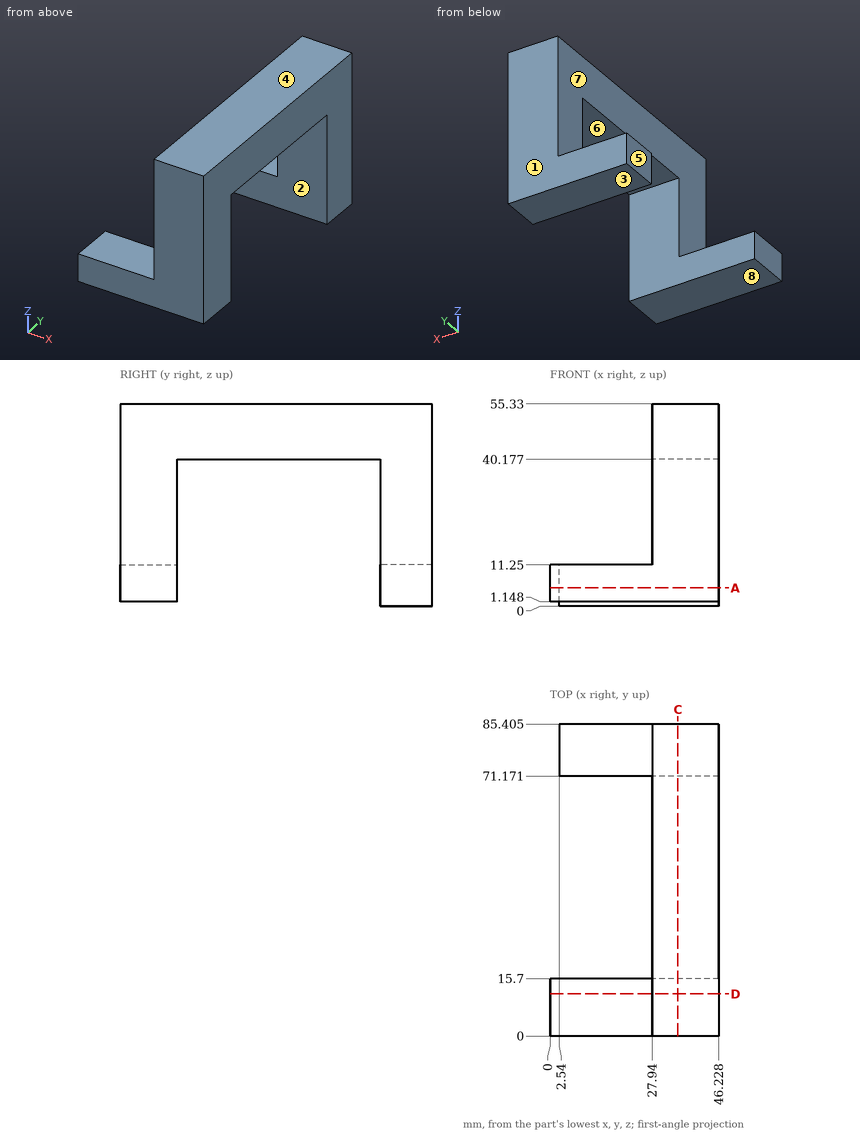
Job drawing, mm, ordinate dimensions from the low corner. One solid piece. A direction names the side the tool comes from. Coordinates: 2 decimals unless noted, no trailing zeros. Loops run counter-clockwise (first coordinate to the right, second up) from the corner with the lowest first, then second, coordinate; pieces in that order, holes last. Notation, with made-up numbers: (48.25, 85) - (89.25, 85) arc R22 cw to (89.25, 102) - close; hole circle Ø3 at (36.25, 69.5). An arc over 180 degrees is marked (long way). Write item = value, one per line. Start each with the question number.
Q1. Cut at A-A, the plane z = 5. List the corners of the cut face in (x, y) (1 decimal), then the cut area to 3 significant figures.
Q2. Cut at D-D, the plane y = 11.5. List the corners of the cut face in (x, z), then the cut area to 3 significant figures.
Q3. Which spindle directions (+Z, -Z, +X, -X, +Y, -Y) get a long thin tool onto all of the face, cutting with end or side? Do the marked faces 4, 5, 6, 7 and 8. Say none if no direction does.
Q4. Cut at C-C, the plane x = 35. List the corners of the cut face in (y, z) (1 decimal).
Q5. Flat gauge pins, fed straight in: pin 1 Ø12.5 at (x, y) = (18.5, 4) entering from -Z; pin 2 Ø5.5 at (x, y) = (40, 51) entering from -Z; pin 3 Ø15.5 at (x, y) = (14.5, 79) entering from +Z. Where does each tip first touch, or does it go through?
Q6. Drill centre lines: L1, parallel to Y at x = 40.5, z = 23.5 (1 decimal); L2, parallel to X at y = 14.5, z = 45; L3, parallel to Z at x = 23.5, y = 8.5. Where is each one in solid material? Low to high.
Q7. Pull direction Y, two halves, no side cores. Call the marked faces 1, 2 and 3: pulls with the +Y half, pulls with the -Y half, needs draft (parallel to the pull), parting line crosses it, or undercut.
Computed:
q1.outline = (0, 0) - (46.2, 0) - (46.2, 15.7) - (0, 15.7) - close; (2.5, 71.2) - (46.2, 71.2) - (46.2, 85.4) - (2.5, 85.4) - close
q1.area = 1,350 mm²
q2.outline = (0, 1.15) - (46.23, 1.15) - (46.23, 55.33) - (27.94, 55.33) - (27.94, 11.25) - (0, 11.25) - close
q2.area = 1,270 mm²
q3.face_4 = +Z, +X, -X, +Y, -Y
q3.face_5 = +Z, -Z, -X, +Y
q3.face_6 = -Z, +X, -X
q3.face_7 = +Z, -X, +Y, -Y
q3.face_8 = -Z, +X, -X, -Y
q4.outline = (0, 1.1) - (15.7, 1.1) - (15.7, 40.2) - (71.2, 40.2) - (71.2, 0) - (85.4, 0) - (85.4, 55.3) - (0, 55.3) - close
q5.pin_1 = 1.15
q5.pin_2 = 40.18
q5.pin_3 = 11.25
q6.L1 = 0 to 15.7, 71.2 to 85.4
q6.L2 = 27.94 to 46.23
q6.L3 = 1.15 to 11.25
q7.face_1 = pulls with the +Y half
q7.face_2 = undercut
q7.face_3 = needs draft
